Could you check a few things on this drawing? It's one solid part, dimensions in mm from its lowest x, y, z. A direction names the side the tool comes from. Coordinates: 2 decimals unless noted, no trailing zeros. Order: outer loops, then holes, each group sorted by start corner. A loop starts at its lowest first (then second) coordinate and runs counter-clockwise, first axis right, second up. Notation, with made-up numbers: (51.25, 43) -> (81.25, 43) arc R31 ccw to (81.25, 72) -> close; hole circle Ø4 at (10.5, -10). An arc over 180 degrees is marked (long way). Answer as CSV lines item,"result".
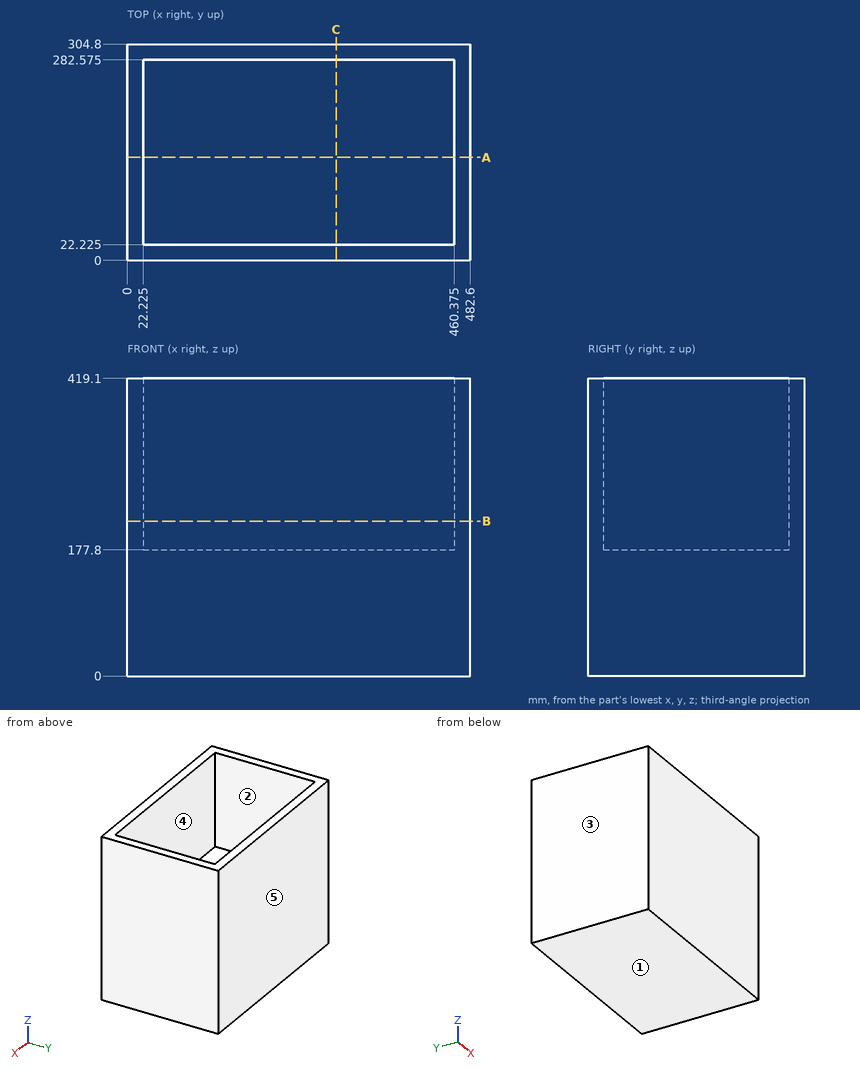
Q1. Imagine slicing it at C-C (x = 294). List the corners of the cut face in (y, z) for me (3 decimals), and give its area (3 significant figures).
Solution:
outline,"(0, 0) -> (304.8, 0) -> (304.8, 419.1) -> (282.575, 419.1) -> (282.575, 177.8) -> (22.225, 177.8) -> (22.225, 419.1) -> (0, 419.1) -> close"
area,"64,900 mm2"
Q2. Imagine slicing it at A-A (y = 145). List the corners of the cut face in (x, z) for me (3 decimals).
Solution:
outline,"(0, 0) -> (482.6, 0) -> (482.6, 419.1) -> (460.375, 419.1) -> (460.375, 177.8) -> (22.225, 177.8) -> (22.225, 419.1) -> (0, 419.1) -> close"
Q3. We'd pull the mould along X, two halves only. Please class the marked faces 3, 4 and 5: pulls with the +X half, pulls with the -X half, needs draft (parallel to the pull), parting line crosses it, or undercut.
Solution:
face 3,"pulls with the -X half"
face 4,"undercut"
face 5,"needs draft"
Q4. For P1, Ø5, axis at x = 102, y = 234.5, coming from the +Z side; P2, Ø5, axis at x = 134, y = 230, coming from the -Z side, each with a flat end and sliding along its axis, tell me the tip position at first contact or that it passes through.
Solution:
P1,"z = 177.8"
P2,"z = 0"
Q5. Which directions (+Z, -Z, +X, -X, +Y, -Y) give clear straight access to the entire face, cutting with the end or side of a thin tool? Please do the marked faces 1 and 2.
Solution:
face 1,"-Z, +X, -X, +Y, -Y"
face 2,"+Z"
Q6. If I drill on line 1 (Y direction, x = 234, z = 374.5) (3 decimals); line 2 (X direction, y = 170.5, z = 393) (3 decimals); line 3 (Z direction, x = 362, y = 186), over which ranges is the centre line in solid material (lowest first)?
Solution:
line 1,"0 to 22.225, 282.575 to 304.8"
line 2,"0 to 22.225, 460.375 to 482.6"
line 3,"0 to 177.8"
Q7. Imagine slicing it at B-B (z = 218). List the corners of the cut face in (x, y) for me (3 decimals), and give its area (3 significant figures).
Solution:
outline,"(0, 0) -> (482.6, 0) -> (482.6, 304.8) -> (0, 304.8) -> close; hole (22.225, 22.225) -> (460.375, 22.225) -> (460.375, 282.575) -> (22.225, 282.575) -> close"
area,"33,000 mm2"
